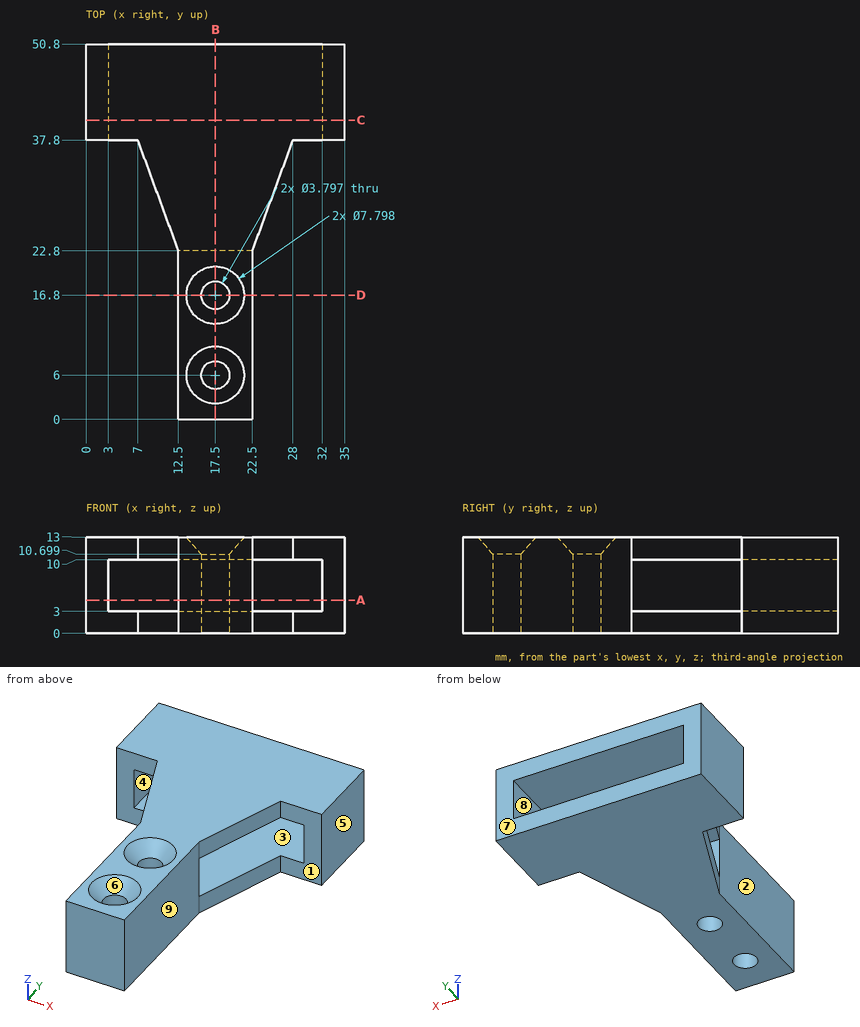
The figure shows three views and two pictorial views of one solid part (mm, origin at its lowest corner). Answer the questions. A direction names the side the tool comes from. Coordinates: 2 decimals unless noted, no trailing zeros. Loops run counter-clockwise (first coordinate to the right, second up) from the corner with the lowest first, then second, coordinate; pieces in that order, holes last.
(1) The mould has two halves that part along X. Classify the marked faces 6, 7, 8 and 9: released by +X, released by -X, zero draft, split by the parting line, or undercut.
Solution:
face 6: undercut
face 7: zero draft
face 8: undercut
face 9: released by +X
(2) The part is cut by section B-B (x = 17.5). Determine the outline of the cut face in (y, z).
Solution:
outline: (0, 0) - (4.1, 0) - (4.1, 10.7) - (2.1, 13) - (0, 13) - close; (7.9, 0) - (14.9, 0) - (14.9, 10.7) - (12.9, 13) - (9.9, 13) - (7.9, 10.7) - close; (18.7, 0) - (50.8, 0) - (50.8, 3) - (22.8, 3) - (22.8, 10) - (50.8, 10) - (50.8, 13) - (20.7, 13) - (18.7, 10.7) - close
(3) The part is cut by section C-C (y = 40.5). Determine the outline of the cut face in (x, z).
Solution:
outline: (0, 0) - (35, 0) - (35, 13) - (0, 13) - close; hole (3, 3) - (32, 3) - (32, 10) - (3, 10) - close
(4) The part is cut by section A-A (z = 4.5). Determine the outline of the cut face in (x, y), and give its area (3 significant figures).
Solution:
outline: (0, 37.8) - (3, 37.8) - (3, 50.8) - (0, 50.8) - close; (12.5, 0) - (22.5, 0) - (22.5, 22.8) - (12.5, 22.8) - close; (32, 37.8) - (35, 37.8) - (35, 50.8) - (32, 50.8) - close; hole circle Ø3.8 at (17.5, 6); hole circle Ø3.8 at (17.5, 16.8)
area: 283 mm2
(5) A tool of negligible diameter and unlimited length cuts with its end or side. For the marked faces 1, 2, 3, 4 and 5, from which of +Z, -Z, +X, -X, +Y, -Y can it reach the whole face along a straight path? Write none if from no direction.
Solution:
face 1: +Z, -Z, +X, -Y
face 2: +Z, -Z, -X, -Y
face 3: +Y
face 4: +Y, -Y
face 5: +Z, -Z, +X, +Y, -Y
(6) The part is cut by section D-D (y = 16.8). Determine the outline of the cut face in (x, z).
Solution:
outline: (12.5, 0) - (15.6, 0) - (15.6, 10.7) - (13.6, 13) - (12.5, 13) - close; (19.4, 0) - (22.5, 0) - (22.5, 13) - (21.4, 13) - (19.4, 10.7) - close
(7) Consider line 1 along Y through (x, z) = (17.5, 4.5); line 2 along X through (y, z) = (46, 9.25); line 3 along Z through (x, y) = (20, 28). Determine where each line is inside the solid, lowest interval first.
Solution:
line 1: y = 0 to 4.1, 7.9 to 14.9, 18.7 to 22.8
line 2: x = 0 to 3, 32 to 35
line 3: z = 0 to 3, 10 to 13
(8) Flat-ended cylindrical pins translate along their axes: pin 1 Ø2 at (x, y) = (10, 5.5) entering from +Z; pin 2 Ø5 at (x, y) = (16.5, 32.5) entering from -Z; pin 3 Ø6.5 at (y, z) = (12.5, 7) entering from +X; pin 4 Ø6.5 at (y, z) = (13.5, 9) entering from -X. Find the tip coordinate at first contact, or state that the pin passes through.
Solution:
pin 1: passes through
pin 2: stops at z = 0
pin 3: stops at x = 22.5
pin 4: stops at x = 12.5
